```python
from build123d import *

# Parameters (mm, degrees)
SKETCH130_R                                        = 19.05
BOSS_EXTRUDE6_DEPTH                                = 20
HEATCARTRIDGEHOLE9_32_0_28125_DIAMETER_D           = 6.1
HEATCARTRIDGEHOLE9_32_0_28125_DIAMETER_DEPTH       = 12
HEATCARTRIDGEHOLE9_32_0_28125_DIAMETER_CSINK_D     = 6.15
HEATCARTRIDGEHOLE9_32_0_28125_DIAMETER_CSINK_ANGLE = 90
HEATCARTRIDGEHOLE9_32_0_28125_DIAMETER_TIP         = 1.832624888
F_2_0_2_DIAMETER_HOLE1_D                           = 2
F_2_0_2_DIAMETER_HOLE1_DEPTH                       = 5
F_2_0_2_DIAMETER_HOLE1_CSINK_D                     = 2.05
F_2_0_2_DIAMETER_HOLE1_CSINK_ANGLE                 = 90
F_2_0_2_DIAMETER_HOLE1_TIP                         = 0.600860619
F_3_0_3_DIAMETER_HOLE1_D                           = 3
F_3_0_3_DIAMETER_HOLE1_DEPTH                       = 5
F_3_0_3_DIAMETER_HOLE1_CSINK_D                     = 3.05
F_3_0_3_DIAMETER_HOLE1_CSINK_ANGLE                 = 90
F_3_0_3_DIAMETER_HOLE1_TIP                         = 0.901290929
F_6_0_6_DIAMETER_HOLE2_D                           = 6
F_6_0_6_DIAMETER_HOLE2_DEPTH                       = 35.197418143
F_6_0_6_DIAMETER_HOLE2_CSINK_D                     = 6.05
F_6_0_6_DIAMETER_HOLE2_CSINK_ANGLE                 = 90
F_6_0_6_DIAMETER_HOLE2_TIP                         = 1.802581857
SKETCH182_R                                        = 10.54735
CUT_EXTRUDE17_DEPTH                                = 13


with BuildPart() as part:
    # Sketch130 → Boss-Extrude6 (new body)
    with BuildSketch(Plane(origin=(0, 0, 0), x_dir=(1, 0, 0), z_dir=(0, 1, 0))):
        with Locations(Location((0, 0, 0), (0, 0, 270))):
            Circle(SKETCH130_R)
    extrude(amount=BOSS_EXTRUDE6_DEPTH)

    # HeatCartridgeHole9/32 (0.28125) Diameter Hole1
    with Locations(Plane(origin=(0, 20, 0), x_dir=(1, 0, 0), z_dir=(0, 1, 0))):
        with Locations((4.480746418, 13.790319486)):
            CounterSinkHole(HEATCARTRIDGEHOLE9_32_0_28125_DIAMETER_D / 2, HEATCARTRIDGEHOLE9_32_0_28125_DIAMETER_CSINK_D / 2, depth=HEATCARTRIDGEHOLE9_32_0_28125_DIAMETER_DEPTH, counter_sink_angle=HEATCARTRIDGEHOLE9_32_0_28125_DIAMETER_CSINK_ANGLE)
            with Locations((0, 0, -(HEATCARTRIDGEHOLE9_32_0_28125_DIAMETER_DEPTH + HEATCARTRIDGEHOLE9_32_0_28125_DIAMETER_TIP / 2))):  # 118° drill point
                Cone(0, HEATCARTRIDGEHOLE9_32_0_28125_DIAMETER_D / 2, HEATCARTRIDGEHOLE9_32_0_28125_DIAMETER_TIP, mode=Mode.SUBTRACT)

    # Ø2.0 (2) Diameter Hole1
    with Locations(Plane(origin=(0, 20, 0), x_dir=(1, 0, 0), z_dir=(0, 1, 0))):
        with Locations((9.358798046, 9.027462242)):
            CounterSinkHole(F_2_0_2_DIAMETER_HOLE1_D / 2, F_2_0_2_DIAMETER_HOLE1_CSINK_D / 2, depth=F_2_0_2_DIAMETER_HOLE1_DEPTH, counter_sink_angle=F_2_0_2_DIAMETER_HOLE1_CSINK_ANGLE)
            with Locations((0, 0, -(F_2_0_2_DIAMETER_HOLE1_DEPTH + F_2_0_2_DIAMETER_HOLE1_TIP / 2))):  # 118° drill point
                Cone(0, F_2_0_2_DIAMETER_HOLE1_D / 2, F_2_0_2_DIAMETER_HOLE1_TIP, mode=Mode.SUBTRACT)

    # Ø3.0 (3) Diameter Hole1
    with Locations(Plane(origin=(0, 20, 0), x_dir=(1, 0, 0), z_dir=(0, 1, 0))):
        with Locations((11.691342951, 6.75)):
            CounterSinkHole(F_3_0_3_DIAMETER_HOLE1_D / 2, F_3_0_3_DIAMETER_HOLE1_CSINK_D / 2, depth=F_3_0_3_DIAMETER_HOLE1_DEPTH, counter_sink_angle=F_3_0_3_DIAMETER_HOLE1_CSINK_ANGLE)
            with Locations((0, 0, -(F_3_0_3_DIAMETER_HOLE1_DEPTH + F_3_0_3_DIAMETER_HOLE1_TIP / 2))):  # 118° drill point
                Cone(0, F_3_0_3_DIAMETER_HOLE1_D / 2, F_3_0_3_DIAMETER_HOLE1_TIP, mode=Mode.SUBTRACT)

    # Ø6.0 (6) Diameter Hole2
    with Locations(Plane(origin=(0, 0, 0), x_dir=(-1, 0, 0), z_dir=(0, -1, 0))):
        with Locations((0.946159788, -1.351256215)):
            CounterSinkHole(F_6_0_6_DIAMETER_HOLE2_D / 2, F_6_0_6_DIAMETER_HOLE2_CSINK_D / 2, depth=F_6_0_6_DIAMETER_HOLE2_DEPTH, counter_sink_angle=F_6_0_6_DIAMETER_HOLE2_CSINK_ANGLE)
            with Locations((0, 0, -(F_6_0_6_DIAMETER_HOLE2_DEPTH + F_6_0_6_DIAMETER_HOLE2_TIP / 2))):  # 118° drill point
                Cone(0, F_6_0_6_DIAMETER_HOLE2_D / 2, F_6_0_6_DIAMETER_HOLE2_TIP, mode=Mode.SUBTRACT)

    # Sketch182 → Cut-Extrude17 (cut)
    with BuildSketch(Plane(origin=(0, 20, 0), x_dir=(1, 0, 0), z_dir=(0, 1, 0))):
        with Locations(Location((-0.946159788, -1.351256215, 0), (0, 0, 270))):
            Circle(SKETCH182_R)
    extrude(amount=-CUT_EXTRUDE17_DEPTH, mode=Mode.SUBTRACT)


solid = part.part
```
Work out the finished part from the listing and answer in its coordinate system (mm). A direction names the side the tool comes from. Coordinates: 2 decimals unless noted, no trailing zeros. Write each loop counter-clockwise with the first axis right and the second up, starting at its lowest first coordinate (ties: lowest second). Pieces come first, ordered by that corner, then holes.
Q1. Find the intervals of material crossed by line 1 (Z direction, x = 6, y = 11) (3 decimals); line 2 (Z direction, x = 8.5, y = 18.5); line 3 (X direction, y = 11.5, z = 4), in increasing order.
Q2. Each of these flat-tipped pins is pushed along its axis until it touches: pin 1 Ø12.5 at (x, z) = (-0.95, 1.35) entering from -Y; pin 2 Ø2.5 at (x, z) = (11.69, -6.75) entering from +Y; pin 3 Ø4 at (x, y) = (-8, 8.5) entering from +Z; pin 4 Ø8 at (x, y) = (12, 5) entering from -Z. Where does it stop, or does it pass through?
Q3. A cutting plane is placed at C-C, the plane y = 3.75. Give the vertices of the cut face in (x, z), then the cut area to 3 significant figures.
Q4. A cutting plane is placed at D-D, the plane y = 10. Give the vertices of the cut face in (x, z).
Q5. Which of the six approach directions +Z, -Z, +X, -X, +Y, -Y give full straight-line access (tool end or side, diameter ignored) to faces 1 (the face through (-4, 0, 0)), 2 (the face through (4.878, 13.904, -16.814))?
Q6. A cutting plane is placed at B-B, the plane x = -11. Give the vertices of the cut face in (y, z).
Q7. A cutting plane is placed at A-A, the plane z = 9. Give the vertices of the cut face in (x, y).
Q8. Determine the mould class of faces 3 (the face through (-11.59, 9.86, -15.12)), 4 (the face through (13.19, 17.45, -6.82)), 5 (the face through (9, 20, -5)), 6 (the face through (8.435, 17.453, -8.644)) for opening direction X: released by +X, released by -X, zero draft, split by the parting line, or undercut.
Findings below:
1. line 1: z = -18.08 to -16.435, -11.146 to -6.586, 9.288 to 18.08
1. line 2: z = -17.05 to -9.54, -8.52 to -3.34, 6.04 to 17.05
1. line 3: x = -18.63 to -11.16, 9.26 to 18.63
2. pin 1: stops at y = 0
2. pin 2: stops at y = 14.85
2. pin 3: stops at z = 18.08
2. pin 4: stops at z = -17.29
3. outline: circle Ø38.1 at (0, 0); hole circle Ø6 at (-0.95, 1.35)
3. area: 1,110 mm2
4. outline: circle Ø38.1 at (0, 0); hole circle Ø21.09 at (-0.95, 1.35); hole circle Ø6.1 at (4.48, -13.79)
5. face 1: +Z, -Z, +X, -X, -Y
5. face 2: +Y
6. outline: (0, -15.55) - (20, -15.55) - (20, -1.84) - (7, -1.84) - (7, 4.54) - (20, 4.54) - (20, 15.55) - (0, 15.55) - close
7. outline: (-16.79, 0) - (16.79, 0) - (16.79, 20) - (6.32, 20) - (6.32, 7) - (-8.21, 7) - (-8.21, 20) - (-16.79, 20) - close
8. face 3: split by the parting line
8. face 4: undercut
8. face 5: zero draft
8. face 6: undercut
